from build123d import *

# Parameters (mm, degrees)
SKIZZE6_W                        = 105
SKIZZE6_H                        = 90
AUFSATZ_LINEAR_AUSTRAGEN3_DEPTH  = 15
SKIZZE7_W                        = 98
SKIZZE7_H                        = 83
SCHNITT_LINEAR_AUSTRAGEN1_DEPTH  = 13
SKIZZE8_W                        = 93
SKIZZE8_H                        = 66
SCHNITT_LINEAR_AUSTRAGEN2_DEPTH  = 13
SKIZZE12_W                       = 83
SKIZZE12_H                       = 1
AUFSATZ_LINEAR_AUSTRAGEN4_DEPTH  = 2
SKIZZE13_W                       = 3
SKIZZE13_H                       = 80
SKIZZE13_H_2                     = 3
SKIZZE13_W_2                     = 95
AUFSATZ_LINEAR_AUSTRAGEN5_DEPTH  = 13
SKIZZE14_W                       = 105
SKIZZE14_H                       = 19
AUFSATZ_LINEAR_AUSTRAGEN7_DEPTH  = 2
SKIZZE15_W                       = 105
SKIZZE15_H                       = 12
AUFSATZ_LINEAR_AUSTRAGEN8_DEPTH  = 13
AUFSATZ_LINEAR_AUSTRAGEN13_DEPTH = 7
AUFSATZ_LINEAR_AUSTRAGEN14_DEPTH = 88
SKIZZE28_R                       = 1.25
SCHNITT_LINEAR_AUSTRAGEN3_DEPTH  = 2
VERRUNDUNG1_R                    = 10


with BuildPart() as part:
    # Skizze6 → Aufsatz-Linear austragen3 (new body)
    with BuildSketch(Plane(origin=(0, 0, 0), x_dir=(1, 0, 0), z_dir=(0, 1, 0))):
        with Locations((52.5, 45)):
            Rectangle(SKIZZE6_W, SKIZZE6_H)
    extrude(amount=AUFSATZ_LINEAR_AUSTRAGEN3_DEPTH)

    # Skizze7 → Schnitt-Linear austragen1 (cut)
    with BuildSketch(Plane(origin=(0, 15, 0), x_dir=(1, 0, 0), z_dir=(0, 1, 0))):
        with Locations((52, 45.5)):
            Rectangle(SKIZZE7_W, SKIZZE7_H)
    extrude(amount=-SCHNITT_LINEAR_AUSTRAGEN1_DEPTH, mode=Mode.SUBTRACT)

    # Skizze8 → Schnitt-Linear austragen2 (cut)
    with BuildSketch(Plane(origin=(0, 2, 0), x_dir=(1, 0, 0), z_dir=(0, 1, 0))):
        with Locations((52, 51)):
            Rectangle(SKIZZE8_W, SKIZZE8_H)
    extrude(amount=-SCHNITT_LINEAR_AUSTRAGEN2_DEPTH, mode=Mode.SUBTRACT)

    # Skizze12 → Aufsatz-Linear austragen4 (add)
    with BuildSketch(Plane.XZ):
        Polygon((5.5, -18), (5.5, -84), (12.5, -84), (12.5, -83), (12.5, -19), (12.5, -18), align=None)
        Polygon((95.5, -83), (95.5, -84), (98.5, -84), (98.5, -18), (95.5, -18), (95.5, -19), align=None)
        with Locations((54, -83.5)):
            Rectangle(SKIZZE12_W, SKIZZE12_H)
        with Locations((54, -18.5)):
            Rectangle(SKIZZE12_W, SKIZZE12_H)
    extrude(amount=-AUFSATZ_LINEAR_AUSTRAGEN4_DEPTH)

    # Skizze13 → Aufsatz-Linear austragen5 (add)
    with BuildSketch(Plane(origin=(0, 2, 0), x_dir=(1, 0, 0), z_dir=(0, 1, 0))):
        with Locations((4.5, 47)):
            Rectangle(SKIZZE13_W, SKIZZE13_H)
        with Locations((4.5, 5.5)):
            Rectangle(SKIZZE13_W, SKIZZE13_H_2)
        with Locations((53.5, 5.5)):
            Rectangle(SKIZZE13_W_2, SKIZZE13_H_2)
    extrude(amount=AUFSATZ_LINEAR_AUSTRAGEN5_DEPTH)

    # Skizze14 → Aufsatz-Linear austragen7 (add)
    with BuildSketch(Plane.XZ):
        with Locations((52.5, -92.5)):
            Rectangle(SKIZZE14_W, SKIZZE14_H)
    extrude(amount=-AUFSATZ_LINEAR_AUSTRAGEN7_DEPTH)

    # Skizze15 → Aufsatz-Linear austragen8 (add)
    with BuildSketch(Plane(origin=(0, 2, 0), x_dir=(1, 0, 0), z_dir=(0, 1, 0))):
        with Locations((52.5, 96)):
            Rectangle(SKIZZE15_W, SKIZZE15_H)
    extrude(amount=AUFSATZ_LINEAR_AUSTRAGEN8_DEPTH)

    # Skizze21 → Aufsatz-Linear austragen13 (add)
    with BuildSketch(Plane.XY):
        Polygon((113.660254038, 0), (105, 15), (88.660254038, 43.301270189), (80, 38.301270189), (102.113248654, 0), align=None)
    aufsatz_linear_austragen13 = extrude(amount=-AUFSATZ_LINEAR_AUSTRAGEN13_DEPTH)

    # Spiegeln2: Aufsatz-Linear austragen13 across plane
    add(aufsatz_linear_austragen13.mirror(Plane(origin=(0, 0, -51), x_dir=(1, 0, 0), z_dir=(0, 0, -1))))

    # Skizze22 → Aufsatz-Linear austragen14 (add)
    with BuildSketch(Plane(origin=(0, 0, -7), x_dir=(-1, 0, 0), z_dir=(0, 0, -1))):
        Polygon((-113.660254038, 0), (-105, 0), (-105, 15), align=None)
    extrude(amount=AUFSATZ_LINEAR_AUSTRAGEN14_DEPTH)

    # Skizze28 → Schnitt-Linear austragen3 (cut)
    with BuildSketch(Plane.XZ):
        with Locations(Location((11.322239977, -4.765490033, 0), (0, 0, 270))):
            Circle(SKIZZE28_R)
        with Locations(Location((31.667742372, -3.316351302, 0), (0, 0, 270))):
            Circle(SKIZZE28_R)
        with Locations(Location((64.25520832, -4.765490033, 0), (0, 0, 270))):
            Circle(SKIZZE28_R)
        with Locations(Location((95.104906067, -3.316351302, 0), (0, 0, 270))):
            Circle(SKIZZE28_R)
        with Locations(Location((95.104906067, -98.683648698, 0), (0, 0, 90))):
            Circle(SKIZZE28_R)
        with Locations(Location((64.25520832, -97.234509967, 0), (0, 0, 90))):
            Circle(SKIZZE28_R)
        with Locations(Location((31.667742372, -98.683648698, 0), (0, 0, 90))):
            Circle(SKIZZE28_R)
        with Locations(Location((11.322239977, -97.234509967, 0), (0, 0, 90))):
            Circle(SKIZZE28_R)
        with Locations(Location((108.821722726, -16.067904783, 0), (0, 0, 270))):
            Circle(SKIZZE28_R)
        with Locations(Location((108.821722726, -78.302664898, 0), (0, 0, 270))):
            Circle(SKIZZE28_R)
        with Locations(Location((110.246680606, -50.827682844, 0), (0, 0, 270))):
            Circle(SKIZZE28_R)
        with Locations(Location((2.746653242, -50.827682844, 0), (0, 0, 270))):
            Circle(SKIZZE28_R)
        with Locations(Location((3.570883833, -21.880288219, 0), (0, 0, 270))):
            Circle(SKIZZE28_R)
        with Locations(Location((3.186977763, -79.047966594, 0), (0, 0, 270))):
            Circle(SKIZZE28_R)
    extrude(amount=-SCHNITT_LINEAR_AUSTRAGEN3_DEPTH, mode=Mode.SUBTRACT)

    # Verrundung1
    verrundung1_edges = [part.edges().sort_by_distance(p)[0] for p in [
        (0, 7.5, -102),
        (0, 7.5, 0),
    ]]
    fillet(verrundung1_edges, radius=VERRUNDUNG1_R)


solid = part.part
Check sheet for the modelled part. Datum: model origin and axes. Units: mm. A direction names the side the tool comes from. Give positions to 0.01 mm unless a question says otherwise; leave off trailing zeros. Loops run counter-clockwise (first coordinate to the right, second up) from the corner with the lowest first, then second, coordinate; pieces in that order, holes last. Notation, with made-up numbers: M -4.75,-34 L 4.25,-34 A33 ccw 4.25,-6 Z; hole C 38.25,-34.75 d4. An arc over 180 degrees is marked long. Answer as a JSON object with one key per item and string values. Group by question number.
Q1. Cross-section at B-B on z = -75. Record the cut outline in (x, y), then the cut area to 3 significant figures.
Q2. Cross-section at C-C on y = 29.5. Record the cut outline in (x, z).
Q3. Go/stop test with flat-tipped pins: P1, Ø0.8, axis at x = 4, z = -22, coming from the -Y side; P2, Ø12, axis at x = 21, y = 22, coming from the +Z side. Record where each tip stops, or that it passes through.
Q4. Cross-section at D-D on y = 4.5. Record the cut outline in (x, z).
Q5. Material ranges on line 1 along Z through (x, y) = (37, 11); line 2 along Y through (x, z) = (27.5, -5); line 3 along X through (y, z) = (10.5, -23), recorded low to high. Write a range as [from, to].
Q6. Access from +Z, -Z, +X, -X, +Y, -Y to the whole of each face (thin tool, end or side, straight path). Record for faces 1 (the flat face through (11, 2, -97)), 2 (the flat face through (86.632, 26.814, -98.549)), 3 (the cylindrical face through (3.01, 7.4, -99.15)).
Q7. Cross-section at A-A on x = 70. Record the cut outline in (y, z).
Q8. Release check for a two-part mould opening along X. For faces 4 (the flat face through (61, 12, 0)), 5 (the flat face through (53, 9, -87)), 6 (the flat face through (0, 7, -50)), 7 (the cylindrical face through (10.562, 0.986, -3.774)) record: released by +X, released by -X, zero draft, split by the parting line, or undercut.
Evaluation:
{
 "1": {"outline": "M 0,0 L 12.5,0 L 12.5,2 L 6,2 L 6,15 L 0,15 Z; M 95.5,0 L 113.66,0 L 105,15 L 101,15 L 101,2 L 95.5,2 Z", "area": "239 mm2"},
 "2": {"outline": "M 85.08,-102 L 96.63,-102 L 96.63,-95 L 85.08,-95 Z; M 85.08,-7 L 96.63,-7 L 96.63,0 L 85.08,0 Z"},
 "3": {"P1": "stops at y = 2", "P2": "passes through"},
 "4": {"outline": "M 0,-92 A10 ccw 10,-102 L 111.06,-102 L 111.06,0 L 10,0 A10 ccw 0,-10 Z; hole M 6,-87 L 101,-87 L 101,-7 L 6,-7 Z"},
 "5": {"line 1": "z = [-102, -87], [-7, 0]", "line 2": "y = [0, 15]", "line 3": "x = [0, 6], [101, 107.6]"},
 "6": {"face 1": "-Y", "face 2": "+Z, -Z, -X", "face 3": "-Z, -X, +Y, -Y"},
 "7": {"outline": "M 0,-102 L 15,-102 L 15,-87 L 2,-87 L 2,-83 L 0,-83 Z; M 0,-19 L 2,-19 L 2,-7 L 15,-7 L 15,0 L 0,0 Z"},
 "8": {"face 4": "zero draft", "face 5": "undercut", "face 6": "released by -X", "face 7": "undercut"}
}
